from build123d import *

# Parameters (mm, degrees)
BOSS_EXTRUDE1_DEPTH = 200
SKETCH2_R           = 5
CUT_EXTRUDE1_DEPTH  = 244.385010939


with BuildPart() as part:
    # Sketch1 → Boss-Extrude1 (new body)
    with BuildSketch(Plane(origin=(0, 0, 0), x_dir=(1, 0, 0), z_dir=(0, 1, 0))):
        Polygon((-12.174757282, 0), (17.825242718, 0), (17.825242718, -6), (-132.174757282, -6), (-132.174757282, 0), (-102.174757282, 0), (-102.174757282, 6), (-138.174757282, 6), (-138.174757282, -12), (23.825242718, -12), (23.825242718, 6), (-12.174757282, 6), align=None)
    extrude(amount=BOSS_EXTRUDE1_DEPTH)

    # Sketch2 → Cut-Extrude1 (cut, through all)
    with BuildSketch(Plane(origin=(0, 0, 6), x_dir=(-1, 0, 0), z_dir=(0, 0, -1))):
        with Locations((24.274757282, 100)):
            Circle(SKETCH2_R)
        with Locations(Location((90.074757282, 100, 0), (0, 0, 180))):
            Circle(SKETCH2_R)
    extrude(amount=-CUT_EXTRUDE1_DEPTH, mode=Mode.SUBTRACT)


solid = part.part
Here's how the part is built. I have some questions about the finished solid (model axes, mm). A direction names the side the tool comes from. Give positions to 0.01 mm unless a question says otherwise; leave off trailing zeros. Loops run counter-clockwise (first coordinate to the right, second up) from the corner with the lowest first, then second, coordinate; pieces in that order, holes last. Notation, with made-up numbers: (-21, 41) -> (24, 41) arc R31 ccw to (24, 65) -> close; hole circle Ø10 at (68, 7.25). An arc over 180 degrees is marked (long way). Answer as a JSON object with one key per item and string values. Group by question number.
Item 1: Will these pins go through, and if not, where does the flat tip stop? pin 1 (6 mm diameter, centred on x = -90.07, y = 100, fed in from +Z); pin 2 (11.5 mm diameter, centred on x = -24.27, y = 100, fed in from -Z).
Item 2: Imagine slicing it at B-B on y = 100. Write out the boundary of the cut face in (x, z), then the cut area to 3 significant figures.
Item 3: Imagine slicing it at C-C on y = 138. Write out the boundary of the cut face in (x, z).
Item 4: Thinking about a two-plate mould opening in Z: for faces 4 (the flat face through (-58, 99, 12)), 5 (the flat face through (17.825, 99, 3)), 6 (the flat face through (-138.175, 99, 3)), 7 (the flat face through (-132.175, 99, 3)), which applies, pulls with the +Z half, pulls with the -Z half, needs draft (parallel to the pull), parting line crosses it, or undercut?
Item 5: I need wall thicknesses on L1, parallel to X at y = 12, z = 2.5; L2, parallel to X at y = 100, z = -4.25; L3, parallel to Z at x = -107.5, y = 29.5. Which ranges of each line are inside material? Lowest first, please.
Item 6: Imagine slicing it at D-D on x = -100. Write out the boundary of the cut face in (y, z).
Item 7: Imagine slicing it at A-A on x = -7. Write out the boundary of the cut face in (y, z).
Item 8: On a 3-axis mill with a long thin cutter (end or side, diameter ignored), from which of +Z, -Z, +X, -X, +Y, -Y can I reach the whole of each face in a straight line? I mean faces 1 (the flat face through (-12.175, 99, -3)), 2 (the flat face through (-117, 99, 0)), 3 (the flat face through (23.825, 99, 3)). Say none if no direction works.
Answer list:
{
 "1": {"pin 1": "passes through", "pin 2": "stops at z = 6"},
 "2": {"outline": "(-138.17, -6) -> (-102.17, -6) -> (-102.17, 0) -> (-132.17, 0) -> (-132.17, 6) -> (-95.07, 6) -> (-95.07, 12) -> (-138.17, 12) -> close; (-85.07, 6) -> (-29.27, 6) -> (-29.27, 12) -> (-85.07, 12) -> close; (-19.27, 6) -> (17.83, 6) -> (17.83, 0) -> (-12.17, 0) -> (-12.17, -6) -> (23.83, -6) -> (23.83, 12) -> (-19.27, 12) -> close", "area": "1,360 mm2"},
 "3": {"outline": "(-138.17, -6) -> (-102.17, -6) -> (-102.17, 0) -> (-132.17, 0) -> (-132.17, 6) -> (17.83, 6) -> (17.83, 0) -> (-12.17, 0) -> (-12.17, -6) -> (23.83, -6) -> (23.83, 12) -> (-138.17, 12) -> close"},
 "4": {"face 4": "pulls with the +Z half", "face 5": "undercut", "face 6": "needs draft", "face 7": "undercut"},
 "5": {"L1": "x = -138.17 to -132.17, 17.83 to 23.83", "L2": "x = -138.17 to -102.17, -12.17 to 23.83", "L3": "z = -6 to 0, 6 to 12"},
 "6": {"outline": "(0, 6) -> (200, 6) -> (200, 12) -> (0, 12) -> close"},
 "7": {"outline": "(0, -6) -> (200, -6) -> (200, 0) -> (0, 0) -> close; (0, 6) -> (200, 6) -> (200, 12) -> (0, 12) -> close"},
 "8": {"face 1": "-Z, +Y, -Y", "face 2": "+Y, -Y", "face 3": "+Z, -Z, +X, +Y, -Y"}
}
